The listing builds one solid part. Answer for the finished solid, in the listing's coordinates (mm). A direction names the side the tool comes from. Round coordinates to 2 decimals unless told otherwise and drop trailing zeros. Write each loop counter-clockwise with the first axis right and the second up, starting at its lowest first coordinate (ties: lowest second). Pieces come first, ordered by that corner, then holes.
Item 1: For a pull along X with two mould halves and no side action, classify faces 4 (the face through (17.711, 1.61, -18.205)), 5 (the face through (230, 42.862, -244)), 6 (the face through (254.197, 21.131, -248.667)), 7 (the face through (230.905, 42.058, -236.04)) as +X half, -X half, draft (parallel to the pull), parting line (faces both ways), or undercut.
Item 2: Find section B-B on x = 220.5. Give the vertices of the cut face in (y, z) (1 decimal).
Item 3: Each of these flat-tipped pins is pushed along its axis until it touches: pin 1 (10 mm diameter, centred on x = 238, y = 14.5, fed in from +Z); pin 2 (1.3 mm diameter, centred on x = 354.5, y = 22, fed in from +Z); pin 3 (3.5 mm diameter, centred on x = -64.5, y = 1.5, fed in from -Z); pin 4 (6 mm diameter, centred on x = 229, y = 5.5, fed in from +Z). Where does it stop, or does it pass through?
Item 4: A tool of negligible diameter and unlimited length cuts with its end or side. For faces 1 (the face through (247.56, 21.96, -253.06)), 2 (the face through (26.668, 1.61, 26.707)), 3 (the face through (354.012, 22, 142)), from which of +Z, -Z, +X, -X, +Y, -Y can it reach the whole face along a straight path? Write none if from no direction.
Item 5: Find section C-C on z = -304. Give the vertices of the cut face in (x, y) (1 decimal).
Item 6: Find the intervals of material crossed by probe 1 along Y at (x, z) = (201.5, -289.5) (1 decimal); probe 2 along Y at (x, z) = (318.5, 159) (3 decimals); probe 3 along X at (y, z) = (18.5, 198), in increasing order.
Item 7: Find section A-A on y = 17.5. Give the vertices of the cut face in (x, z) (1 decimal).
Item 8: Find section D-D on z = 229. Give the vertices of the cut face in (x, y) (1 decimal).
```python
from build123d import *

# Parameters (mm, degrees)
BOSS_EXTRUDE1_DEPTH  = 3.175
BOSS_EXTRUDE2_DEPTH  = 38.1
SKETCH4_W            = 1.5875
SKETCH4_H            = 279.4
BOSS_EXTRUDE3_DEPTH  = 38.1
SKETCH6_R            = 1.5875
CUT_EXTRUDE1_DEPTH   = 19.05
SKETCH10_W           = 101.6
SKETCH10_H           = 3.175
BOSS_EXTRUDE5_DEPTH  = 63.5
SKETCH12_W           = 355.6
SKETCH12_H           = 101.6
BOSS_EXTRUDE6_DEPTH  = 3.175
SKETCH13_W           = 63.5
SKETCH13_H           = 63.5
SKETCH13_H_2         = 12.7
BOSS_EXTRUDE7_DEPTH  = 3.175
CUT_EXTRUDE3_DEPTH   = 38.1
BOSS_EXTRUDE10_DEPTH = 1.5875
CUT_EXTRUDE5_DEPTH   = 3.175
SKETCH22_W           = 25.4
SKETCH22_H           = 177.8
BOSS_EXTRUDE11_DEPTH = 3.175
CUT_EXTRUDE6_DEPTH   = 33.02


with BuildPart() as part:
    # Sketch2 → Boss-Extrude1 (new body)
    with BuildSketch(Plane(origin=(0, 0, 0), x_dir=(1, 0, 0), z_dir=(0, 1, 0))):
        with BuildLine():
            Line((0, 355.6), (0, 0))
            Line((0, 0), (0, -304.8))
            Line((0, -304.8), (355.6, -304.8))
            Line((355.6, -304.8), (355.6, 0))
            ThreePointArc((355.6, 0), (251.44717139, 251.44717139), (0, 355.6))
        make_face()
    extrude(amount=BOSS_EXTRUDE1_DEPTH)

    # Sketch3 → Boss-Extrude2 (add)
    with BuildSketch(Plane(origin=(0, 3.175, 0), x_dir=(1, 0, 0), z_dir=(0, 1, 0))):
        with BuildLine():
            Line((0, 355.6), (0, 354.0125))
            ThreePointArc((0, 354.0125), (250.324639375, 250.324639375), (354.0125, 0))
            Line((354.0125, 0), (355.6, 0))
            ThreePointArc((355.6, 0), (251.44717139, 251.44717139), (0, 355.6))
        make_face()
    extrude(amount=BOSS_EXTRUDE2_DEPTH)

    # Sketch4 → Boss-Extrude3 (add)
    with BuildSketch(Plane(origin=(0, 3.175, 0), x_dir=(1, 0, 0), z_dir=(0, 1, 0))):
        with Locations((354.80625, -139.7)):
            Rectangle(SKETCH4_W, SKETCH4_H)
    extrude(amount=BOSS_EXTRUDE3_DEPTH)

    # Sketch6 → Cut-Extrude1 (cut)
    with BuildSketch(Plane(origin=(0, 3.175, 0), x_dir=(1, 0, 0), z_dir=(0, 1, 0))):
        Circle(SKETCH6_R)
    extrude(amount=-CUT_EXTRUDE1_DEPTH, mode=Mode.SUBTRACT)

    # Sketch10 → Boss-Extrude5 (add)
    with BuildSketch(Plane.ZY):
        with Locations((12.7, 1.5875)):
            Rectangle(SKETCH10_W, SKETCH10_H)
    extrude(amount=BOSS_EXTRUDE5_DEPTH)

    # Sketch12 → Boss-Extrude6 (add)
    with BuildSketch(Plane.XZ):
        with Locations((177.8, 355.6)):
            Rectangle(SKETCH12_W, SKETCH12_H)
    extrude(amount=-BOSS_EXTRUDE6_DEPTH)

    # Sketch13 → Boss-Extrude7 (add)
    with BuildSketch(Plane(origin=(0, 3.175, 0), x_dir=(1, 0, 0), z_dir=(0, 1, 0))):
        with Locations((-31.75, 69.85)):
            Rectangle(SKETCH13_W, SKETCH13_H)
        with Locations((-31.75, -69.85)):
            Rectangle(SKETCH13_W, SKETCH13_H_2)
    extrude(amount=-BOSS_EXTRUDE7_DEPTH)

    # Sketch11 → Cut-Extrude3 (cut)
    with BuildSketch(Plane(origin=(0, 3.175, 0), x_dir=(1, 0, 0), z_dir=(0, 1, 0))):
        with BuildLine():
            Line((-22.450640303, 0), (-4.490128061, 17.960512242))
            ThreePointArc((-4.490128061, 17.960512242), (17.960512242, 17.960512242), (17.960512242, -4.490128061))
            Line((17.960512242, -4.490128061), (0, -22.450640303))
            ThreePointArc((0, -22.450640303), (-22.450640303, -22.450640303), (-22.450640303, 0))
        make_face()
    extrude(amount=-CUT_EXTRUDE3_DEPTH, mode=Mode.SUBTRACT)

    # Sketch18 → Boss-Extrude10 (add)
    with BuildSketch(Plane(origin=(0, 41.275, 0), x_dir=(1, 0, 0), z_dir=(0, 1, 0))):
        with BuildLine():
            Line((0, 355.6), (0, 330.2))
            ThreePointArc((0, 330.2), (233.486659148, 233.486659148), (330.2, 0))
            Line((330.2, 0), (355.6, 0))
            ThreePointArc((355.6, 0), (251.44717139, 251.44717139), (0, 355.6))
        make_face()
    extrude(amount=BOSS_EXTRUDE10_DEPTH)

    # Sketch19 → Cut-Extrude5 (cut)
    with BuildSketch(Plane(origin=(44.866081356, 3.175, 35.384906035), x_dir=(-0.707106781186549, 0, -0.7071067811865461), z_dir=(0, 1, 0))):
        with BuildLine():
            Line((19.004203404, 22.579203363), (19.004203404, -9.566550011))
            ThreePointArc((19.004203404, -9.566550011), (13.566017381, -15.004736034), (8.127831358, -9.566550011))
            Line((8.127831358, -9.566550011), (8.127831358, 22.579203363))
            ThreePointArc((8.127831358, 22.579203363), (13.566017381, 28.017389386), (19.004203404, 22.579203363))
        make_face()
        with BuildLine():
            Line((94.473450284, 22.579203363), (94.473450284, -9.566550011))
            ThreePointArc((94.473450284, -9.566550011), (99.926017381, -15.019117108), (105.378584479, -9.566550011))
            Line((105.378584479, -9.566550011), (105.378584479, 22.579203363))
            ThreePointArc((105.378584479, 22.579203363), (99.926017381, 28.03177046), (94.473450284, 22.579203363))
        make_face()
    extrude(amount=-CUT_EXTRUDE5_DEPTH, mode=Mode.SUBTRACT)

    # Sketch22 → Boss-Extrude11 (add)
    with BuildSketch(Plane.XZ):
        with Locations((-76.2, -12.7)):
            Rectangle(SKETCH22_W, SKETCH22_H)
    extrude(amount=-BOSS_EXTRUDE11_DEPTH)

    # Sketch20 → Cut-Extrude6 (cut)
    with BuildSketch(Plane(origin=(269.3998556, -22.225, -80.446532344), x_dir=(1, 0, 0), z_dir=(0, 1, 0))):
        with BuildLine():
            Line((-336.976282911, -51.485206353), (-314.525642608, -29.034566051))
            ThreePointArc((-314.525642608, -29.034566051), (-310.035514547, -29.034566051), (-310.035514547, -33.524694111))
            Line((-310.035514547, -33.524694111), (-332.48615485, -55.975334414))
            ThreePointArc((-332.48615485, -55.975334414), (-336.976282911, -55.975334414), (-336.976282911, -51.485206353))
        make_face()
        with BuildLine():
            Line((-240.438529609, -148.022959655), (-217.987889306, -125.572319352))
            ThreePointArc((-217.987889306, -125.572319352), (-217.987889306, -121.082191292), (-222.478017367, -121.082191292))
            Line((-222.478017367, -121.082191292), (-244.92865767, -143.532831594))
            ThreePointArc((-244.92865767, -143.532831594), (-244.92865767, -148.022959655), (-240.438529609, -148.022959655))
        make_face()
        with BuildLine():
            Line((-249.280873656, -31.417542155), (-226.830233353, -8.966901852))
            ThreePointArc((-226.830233353, -8.966901852), (-222.340105293, -8.966901852), (-222.340105293, -13.457029913))
            Line((-222.340105293, -13.457029913), (-244.790745596, -35.907670216))
            ThreePointArc((-244.790745596, -35.907670216), (-249.280873656, -35.907670216), (-249.280873656, -31.417542155))
        make_face()
        with BuildLine():
            Line((-220.370865411, -60.3275504), (-197.920225108, -37.876910098))
            ThreePointArc((-197.920225108, -37.876910098), (-197.920225108, -33.386782037), (-202.410353169, -33.386782037))
            Line((-202.410353169, -33.386782037), (-224.860993471, -55.83742234))
            ThreePointArc((-224.860993471, -55.83742234), (-224.860993471, -60.3275504), (-220.370865411, -60.3275504))
        make_face()
    extrude(amount=CUT_EXTRUDE6_DEPTH, mode=Mode.SUBTRACT)


solid = part.part
```
Check values:
1. face 4: undercut
1. face 5: draft
1. face 6: +X half
1. face 7: -X half
2. outline: (0, -279) - (42.9, -279) - (42.9, -245.8) - (41.3, -245.8) - (41.3, -277) - (3.2, -277) - (3.2, 406.4) - (0, 406.4) - close
3. pin 1: stops at z = -257.44
3. pin 2: stops at z = 279.4
3. pin 3: stops at z = -101.6
3. pin 4: stops at z = 406.4
4. face 1: +Z, -X
4. face 2: +Y, -Y
4. face 3: +Z, -X, +Y
5. outline: (0, 0) - (184.5, 0) - (184.5, 42.9) - (128.9, 42.9) - (128.9, 41.3) - (181.4, 41.3) - (181.4, 3.2) - (0, 3.2) - close
6. probe 1: y = 0 to 3.2, 41.3 to 42.9
6. probe 2: y = 0 to 3.175
6. probe 3: x = 354.01 to 355.6
7. outline: (0, -355.6) arc R355.6 ccw to (355.6, 0) - (355.6, 279.4) - (354, 279.4) - (354, 0) arc R354 cw to (0, -354) - close
8. outline: (0, 0) - (355.6, 0) - (355.6, 41.3) - (354, 41.3) - (354, 3.2) - (0, 3.2) - close
